from build123d import *

# Parameters (mm, degrees)
BOSS_EXTRUDE1_DEPTH = 254
SKETCH2_R           = 3.3274
CUT_EXTRUDE1_DEPTH  = 260.72974897
SKETCH3_R           = 6.35
CUT_EXTRUDE2_DEPTH  = 12.7


with BuildPart() as part:
    # Sketch1 → Boss-Extrude1 (new body)
    with BuildSketch(Plane.XY):
        with BuildLine():
            Line((-19.05, 0), (19.05, 0))
            Line((19.05, 0), (4.010170085, 26.049749551))
            ThreePointArc((4.010170085, 26.049749551), (0, 50.8), (-4.010170085, 26.049749551))
            Line((-4.010170085, 26.049749551), (-19.05, 0))
        make_face()
    extrude(amount=BOSS_EXTRUDE1_DEPTH)

    # Sketch2 → Cut-Extrude1 (cut, through all)
    with BuildSketch(Plane.XZ):
        with Locations(Location((0, 190.5, 0), (0, 0, 270))):
            Circle(SKETCH2_R)
        with Locations(Location((0, 63.5, 0), (0, 0, 270))):
            Circle(SKETCH2_R)
    extrude(amount=-CUT_EXTRUDE1_DEPTH, mode=Mode.SUBTRACT)

    # Sketch3 → Cut-Extrude2 (cut)
    with BuildSketch(Plane(origin=(0, 50.8, 0), x_dir=(1, 0, 0), z_dir=(0, 1, 0))):
        with Locations(Location((0, -63.5, 0), (0, 0, 270))):
            Circle(SKETCH3_R)
        with Locations(Location((0, -190.5, 0), (0, 0, 270))):
            Circle(SKETCH3_R)
    extrude(amount=-CUT_EXTRUDE2_DEPTH, mode=Mode.SUBTRACT)


solid = part.part
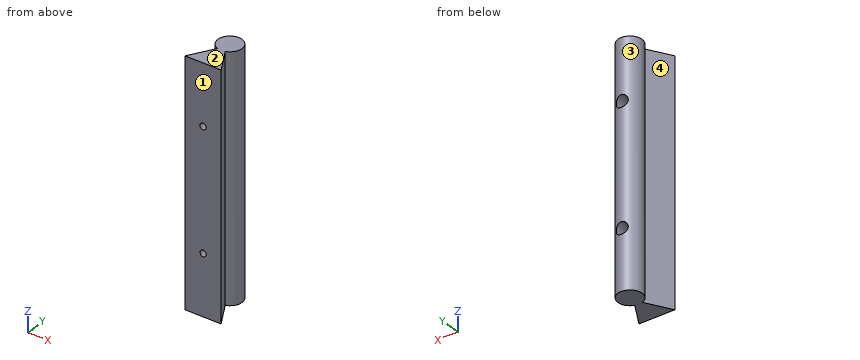
Work out the finished part from the listing and answer in its coordinate system (mm). Face numbers are marked on the shaded views. Round coordinates to 2 decimals unless told otherwise and drop trailing zeros. Write each loop counter-clockwise with the first axis right and the second up, starting at its lowest first coordinate (ties: lowest second). Pieces come first, ordered by that corner, then holes.
1) Straight lines are drawn through the part: line 1 (Z direction, x = 0, y = 48); line 2 (Y direction, x = -9.5, z = 224); line 3 (Y direction, x = 7.5, z = 16.5). For each, find the intervals that lie inside material, in ascending order.
2) A cutting plane is placed at D-D (y = 30). Give the vertices of the cut face in (x, z).
3) The mould has two halves that part along Y. Classify the marked faces 1, 2, 3 and 4: pulls with the +Y half, pulls with the -Y half, needs draft (parallel to the pull), parting line crosses it, or undercut.
4) A cutting plane is placed at C-C (z = 63.5). Give the vertices of the cut face in (x, y), plus the area to 3 significant figures.
5) Given pin 1 Ø7.5 at (x, z) = (0, 63.5) entering from +Y; pin 2 Ø1 at (y, z) = (35.5, 75) entering from -X; pin 3 Ø1 at (y, z) = (20, 152.5) entering from -X, each flat-ended and moving along its own axis, determine where each tip first touches the part or whether it passes through.
6) A cutting plane is placed at B-B (y = 45). Give the vertices of the cut face in (x, z), plus the area to 3 significant figures.
7) A cutting plane is placed at A-A (x = 0). Give the vertices of the cut face in (y, z), plus the area to 3 significant figures.
Completed:
1. line 1: z = 0 to 57.15, 69.85 to 184.15, 196.85 to 254
1. line 2: y = 0 to 16.54, 29.67 to 46.53
1. line 3: y = 0 to 20.01, 27.85 to 48.35
2. outline: (-9.78, 0) - (9.78, 0) - (9.78, 254) - (-9.78, 254) - close; hole circle Ø6.65 at (0, 63.5); hole circle Ø6.65 at (0, 190.5)
3. face 1: pulls with the -Y half
3. face 2: needs draft
3. face 3: undercut
3. face 4: undercut
4. outline: (-19.05, 0) - (-3.33, 0) - (-3.33, 38.1) - (-6.35, 38.1) - (-6.35, 49.1) arc R12.7 ccw to (-4.01, 26.05) - close; (3.33, 0) - (19.05, 0) - (4.01, 26.05) arc R12.7 ccw to (6.35, 49.1) - (6.35, 38.1) - (3.33, 38.1) - close
4. area: 696 mm2
5. pin 1: stops at y = 38.1
5. pin 2: stops at x = -12.53
5. pin 3: stops at x = -7.79
6. outline: (-10.66, 0) - (10.66, 0) - (10.66, 254) - (-10.66, 254) - close; hole circle Ø12.7 at (0, 63.5); hole circle Ø12.7 at (0, 190.5)
6. area: 5,160 mm2
7. outline: (0, 0) - (50.8, 0) - (50.8, 57.15) - (38.1, 57.15) - (38.1, 60.17) - (0, 60.17) - close; (0, 66.83) - (38.1, 66.83) - (38.1, 69.85) - (50.8, 69.85) - (50.8, 184.15) - (38.1, 184.15) - (38.1, 187.17) - (0, 187.17) - close; (0, 193.83) - (38.1, 193.83) - (38.1, 196.85) - (50.8, 196.85) - (50.8, 254) - (0, 254) - close
7. area: 12,100 mm2
